Here's how the part is built. I have some questions about the finished solid (model axes, mm). Face numbers are marked on the shaded views. A direction names the side the tool comes from. Round coordinates to 2 decimals unless told otherwise and drop trailing zeros. Write each loop counter-clockwise with the first axis right and the second up, starting at its lowest first coordinate (ties: lowest second). Pieces come first, ordered by that corner, then holes. Notation, with made-up numbers: (47.25, 32.5) -> (76.25, 32.5) arc R15 ccw to (76.25, 39.5) -> close; hole circle Ø1 at (31, 10.25). An arc over 180 degrees is marked (long way). Answer as CSV lines item,"result".
from build123d import *

# Parameters (mm, degrees)
EXTRUDE_1_DEPTH     = 10
SKETCH_2_R          = 28
EXTRUDE_2_DEPTH     = 50
SKETCH_3_R          = 24
CUT_EXTRUDE_1_DEPTH = 30
SKETCH_4_R          = 10
CUT_EXTRUDE_2_DEPTH = 60


with BuildPart() as part:
    # Эскиз1 → Бобышка-Вытянуть1 (new body)
    with BuildSketch(Plane.XY):
        Polygon((45, 19.166666667), (55, 19.166666667), (50.333333333, 31.166666667), (-50, 31.166666667), (-55, 19.166666667), (-45, 19.166666667), (-40, 0), (-45, -19.166666667), (-55, -19.166666667), (-50, -31.166666667), (50, -31.166666667), (55, -19.166666667), (45, -19.166666667), (40, 0), align=None)
    extrude(amount=EXTRUDE_1_DEPTH)

    # Эскиз2 → Бобышка-Вытянуть2 (add)
    with BuildSketch(Plane.XY.offset(10)):
        Circle(SKETCH_2_R)
    extrude(amount=EXTRUDE_2_DEPTH)

    # Эскиз3 → Вырез-Вытянуть1 (cut)
    with BuildSketch(Plane.XY.offset(60)):
        Circle(SKETCH_3_R)
    extrude(amount=-CUT_EXTRUDE_1_DEPTH, mode=Mode.SUBTRACT)

    # Эскиз4 → Вырез-Вытянуть2 (cut)
    with BuildSketch(Plane.XY.offset(30)):
        Circle(SKETCH_4_R)
    extrude(amount=-CUT_EXTRUDE_2_DEPTH, mode=Mode.SUBTRACT)


solid = part.part
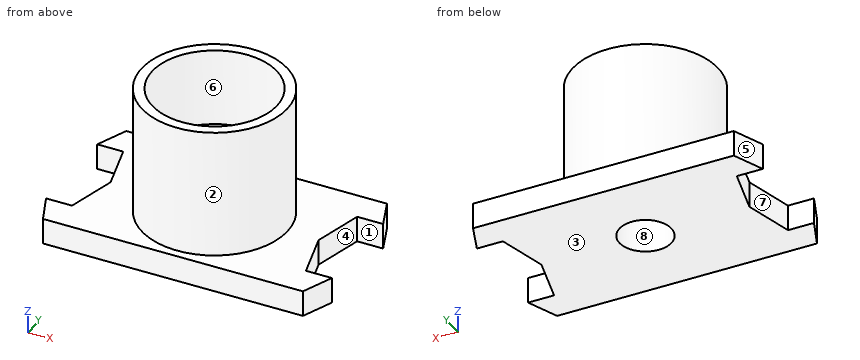
Item 1: If we mould it in two halves opening along Y, with no side actions, what happens to the marked faces 1, 2 and 3? For each: pulls with the +Y half, pulls with the -Y half, needs draft (parallel to the pull), parting line crosses it, or undercut.
Results found:
face 1,"undercut"
face 2,"parting line crosses it"
face 3,"needs draft"
Item 2: Suppose I cut it at C-C, the plane y = 2.5. List the corners of the cut face in (x, z) for me.
Results found:
outline,"(-40.65, 0) -> (-9.68, 0) -> (-9.68, 30) -> (-23.87, 30) -> (-23.87, 60) -> (-27.89, 60) -> (-27.89, 10) -> (-40.65, 10) -> close; (9.68, 0) -> (40.65, 0) -> (40.65, 10) -> (27.89, 10) -> (27.89, 60) -> (23.87, 60) -> (23.87, 30) -> (9.68, 30) -> close"
Item 3: For the marked faces 4, 5, 6, 7 and 8, which set-ups out of +Z, -Z, +X, -X, +Y, -Y let a thin tool reach every point of the face, with its end or its side?
Results found:
face 4,"+Z, -Z, +X"
face 5,"+Z, -Z, -X, +Y"
face 6,"+Z"
face 7,"+Z, -Z, -X"
face 8,"+Z, -Z"
Item 4: I need wall thicknesses on L1, parallel to Y at x = 0, z = 47; L2, parallel to Y at x = 0, z = 19; L3, parallel to Z at x = -45.5, y = -26.5. Which ranges of each line are inside material? Lowest first, please.
Results found:
L1,"y = -28 to -24, 24 to 28"
L2,"y = -28 to -10, 10 to 28"
L3,"z = 0 to 10"
Item 5: Suppose I cut it at B-B, the plane z = 8.5. List the corners of the cut face in (x, y) for me.
Results found:
outline,"(-55, -19.17) -> (-50, -31.17) -> (50, -31.17) -> (55, -19.17) -> (45, -19.17) -> (40, 0) -> (45, 19.17) -> (55, 19.17) -> (50.33, 31.17) -> (-50, 31.17) -> (-55, 19.17) -> (-45, 19.17) -> (-40, 0) -> (-45, -19.17) -> close; hole circle Ø20 at (0, 0)"
Item 6: Suppose I cut it at D-D, the plane x = 0. List the corners of the cut face in (y, z) for me.
Results found:
outline,"(-31.17, 0) -> (-10, 0) -> (-10, 30) -> (-24, 30) -> (-24, 60) -> (-28, 60) -> (-28, 10) -> (-31.17, 10) -> close; (10, 0) -> (31.17, 0) -> (31.17, 10) -> (28, 10) -> (28, 60) -> (24, 60) -> (24, 30) -> (10, 30) -> close"
Item 7: Will these pins go through, and if not, where does the flat tip stop? pin 1 (2 mm diameter, centred on y = 3, z = 27, fed in from +X); pin 2 (16 mm diameter, centred on x = 0, y = 0, fed in from +Z); pin 3 (6 mm diameter, centred on y = 14, z = 22, fed in from +X); pin 4 (1 mm diameter, centred on y = -7.5, z = 27, fed in from -X).
Results found:
pin 1,"stops at x = 27.93"
pin 2,"passes through"
pin 3,"stops at x = 25.75"
pin 4,"stops at x = -27.11"
Item 8: Suppose I cut it at A-A, the plane x = -47. List the corners of the cut face in (y, z) for me, then the cut area to 3 significant figures.
Results found:
outline,"(-31.17, 0) -> (-19.17, 0) -> (-19.17, 10) -> (-31.17, 10) -> close; (19.17, 0) -> (31.17, 0) -> (31.17, 10) -> (19.17, 10) -> close"
area,"240 mm²"
